Input: part model. Units: mm. Frame: model coordinates. A direction names the side the tool comes from. Round coordinates to 2 decimals unless told otherwise and drop trailing zeros. Write each loop counter-clockwise with the first axis right and the second up, starting at its lowest first coordinate (ties: lowest second). Pieces come first, ordered by that corner, then holes. Notation, with made-up numbers: (-18, 67) - (1, 67) arc R24 ccw to (1, 102) - close; hole circle Ø9 at (64, 51). An arc over 180 degrees is marked (long way). One line per item, written item: value. Start each with the question number.
Autodesk Inventor part; units mm, degrees
ref_plane "YZ Plane" through (0, 0, 0) normal (1, 0, 0) x (0, 1, 0)
ref_plane "XZ Plane" through (0, 0, 0) normal (0, 1, 0) x (-1, 0, 0)
ref_plane "XY Plane" through (0, 0, 0) normal (0, 0, 1) x (1, 0, 0)
sketch "Sketch1" plane through (0, 0, 0) normal (0, 1, 0) x (-1, 0, 0)
  point P0 (0, 0)
sketch "Sketch2" plane through (0, 0, 0) normal (0, 1, 0) x (-1, 0, 0)
  circle A0 centre (0, 0) radius 2
  dimension "d0" = 4
extrude "Extrusion1" add sketch "Sketch2" along normal blind 51
sketch "Sketch3" plane through (0, 0, 0) normal (0, -1, 0) x (1, 0, 0)
  line L0 (-0.5, 2) -> (0.5, 2)
  line L1 (0.5, 2) -> (0.5, -2)
  line L2 (0.5, -2) -> (-0.5, -2)
  line L3 (-0.5, -2) -> (-0.5, 2)
  line L4 (-0.5, 2) -> (0.5, -2) construction
  line L5 (0.5, 2) -> (-0.5, -2) construction
  point P0 (0, 0)
  dimension "d3" = 1
  dimension "d4" = 4
extrude "Extrusion2" cut sketch "Sketch3" against normal blind 4
sketch "Sketch4" plane through (0, 51, 0) normal (0, 1, 0) x (1, 0, 0)
  line L0 (0, 9.5) -> (0, -9.5) construction
  line L1 (9.5, 0) -> (-9.5, 0) construction
  line L2 (9.5, 0) -> (9.3816, 1.4953)
  line L3 (9.3816, 1.4953) -> (5.8107, 1.4953)
  line L4 (9.5, 0) -> (9.3816, -1.4953)
  line L5 (9.3816, -1.4953) -> (5.8107, -1.4953)
  line L6 (1.4882, -5.8125) -> (1.4882, -9.3827)
  line L7 (-1.4882, -5.8125) -> (-1.4882, -9.3827)
  line L8 (1.4882, 5.8125) -> (1.4882, 9.3827)
  line L9 (-1.4882, 5.8125) -> (-1.4882, 9.3827)
  line L10 (7.659, -5.6204) -> (4.9964, -3.322)
  line L11 (7.659, -5.6204) -> (6.6789, -6.7559)
  line L12 (6.6789, -6.7559) -> (5.5323, -7.723)
  line L13 (5.5323, -7.723) -> (2.7851, -5.3144)
  line L14 (7.659, 5.6204) -> (4.9964, 3.322)
  line L15 (5.5323, 7.723) -> (2.7851, 5.3144)
  line L16 (-9.5, 0) -> (-9.5, 5) construction
  line L17 (-9.5, 0) -> (-9.5, -5) construction
  line L18 (-8.0777, 5) -> (-3.0777, 5)
  line L19 (-8.0777, -5) -> (-3.0777, -5)
  line L20 (-1.4882, 5.8125) -> (-3.0777, 5)
  line L21 (-3.0777, -5) -> (-1.4882, -5.8125)
  arc A0 (-8.0777, 5) -> (-8.0777, -5) centre (0, 0) ccw
  arc A1 (-1.4882, -9.3827) -> (1.4882, -9.3827) centre (0, 0) ccw
  arc A2 (5.5323, -7.723) -> (7.659, -5.6204) centre (0, 0) ccw
  arc A3 (9.3816, -1.4953) -> (9.3816, 1.4953) centre (0, 0) ccw
  arc A4 (7.659, 5.6204) -> (5.5323, 7.723) centre (0, 0) ccw
  arc A5 (1.4882, 9.3827) -> (-1.4882, 9.3827) centre (0, 0) ccw
  arc A6 (5.8107, 1.4953) -> (4.9964, 3.322) centre (0, 0) ccw
  arc A7 (4.9964, -3.322) -> (5.8107, -1.4953) centre (0, 0) ccw
  arc A8 (1.4882, -5.8125) -> (2.7851, -5.3144) centre (0, 0) ccw
  arc A9 (2.7851, 5.3144) -> (1.4882, 5.8125) centre (0, 0) ccw
  dimension "d28" = 5
  dimension "d29" = 5
extrude "Extrusion3" add sketch "Sketch4" along normal blind 1 contours L4 L5 A7 L10 L11 L12 L13 A8 L6 A1 L7 L21 L19 A0 L18 L20 L9 A5 L8 A9 L15 A4 L14 A6 L3 L2
fillet "Fillet1" radius 1.4 10 edges at (1.4882, 51.5, 9.3827) (-1.4882, 51.5, 9.3827) (9.3816, 51.5, 1.4953) (9.3816, 51.5, -1.4953) (7.659, 51.5, -5.6204) (5.5323, 51.5, -7.723) (1.4882, 51.5, -9.3827) (-1.4882, 51.5, -9.3827) (5.5323, 51.5, 7.723) (7.659, 51.5, 5.6204)
sketch "Sketch5" plane through (0, 52, 0) normal (0, 1, 0) x (1, 0, 0)
  circle A0 centre (0, 0) radius 2
  dimension "d33" = 4
extrude "Extrusion4" add sketch "Sketch5" along normal blind 7
properties part number "Main turning shaft"
Q1. Cut plane B-B, the plane x = -4.75. Output: boundary loops of the cut face in (y, z).
Q2. Cut plane C-C, the plane y = 36.5. Output: boundary loops of the cut face in (x, z), and give its area (3 significant figures).
Q3. Cut plane A-A, the plane z = 0.75. Output: boundary loops of the cut face in (x, y).
Q4. Access query for faces 1 (the flat face through (-0.5, 2, 0)), 2 (the cylindrical face through (2.16, 51.493, 5.598)), 3 (the flat face through (3.725, 51.493, -6.139)), 4 (the flat face through (-2.2, 52, -0.1)). Directions: +Z, -Z, +X, -X, +Y, -Y. A direction counts if a zero-diameter tool reaches every point of the face in a straight line with its end or side. Return the directions, or none.
Q5. Contact query for flat-ended pins moving along their axis: pin 1 Ø0.5 at (x, y) = (-5.5, 51.5) entering from +Z; pin 2 Ø0.8 at (y, z) = (51.5, 6.5) entering from +X; pin 3 Ø0.5 at (x, y) = (6.5, 51.5) entering from +Z. Output: stop coordinate, or through.
Q6. Material intervals for probe 1 along Y at (x, z) = (3, 4); probe 2 along X at (y, z) = (3, -1); probe 3 along X at (y, z) = (38.5, -1), sorted ascending. Write a range as from..to.
Q7. Pull-direction query (Z, two-part tool) for faces 5 (the cylindrical face through (5.5, 51.5, 2.4)), 6 (the cylindrical face through (1.094, 51.507, -9.073)), 7 (the cylindrical face through (5.474, 51.493, -2.456)), 8 (the flat face through (0, 59, 0)); classes: pulls with the +Z half, pulls with the -Z half, needs draft (parallel to the pull), parting line crosses it, or undercut.
A:
1. outline: (51, -5) - (52, -5) - (52, 5) - (51, 5) - close
2. outline: circle Ø4 at (0, 0)
2. area: 12.6 mm²
3. outline: (-9.47, 51) - (-1.85, 51) - (-1.85, 0) - (-0.5, 0) - (-0.5, 4) - (0.5, 4) - (0.5, 0) - (1.85, 0) - (1.85, 51) - (9.33, 51) - (9.33, 52) - (1.85, 52) - (1.85, 59) - (-1.85, 59) - (-1.85, 52) - (-9.47, 52) - close
4. face 1: +Z, -Z, -Y
4. face 2: +Z, +Y, -Y
4. face 3: -Z, +Y, -Y
4. face 4: +Y
5. pin 1: stops at z = 5
5. pin 2: stops at x = 7.04
5. pin 3: stops at z = 7.09
6. probe 1: y = 51..52
6. probe 2: x = -1.73..-0.5, 0.5..1.73
6. probe 3: x = -1.73..1.73
7. face 5: undercut
7. face 6: pulls with the -Z half
7. face 7: undercut
7. face 8: needs draft
